from build123d import *

# Parameters (mm, degrees)
F0_R     = 1.5
F1_DEPTH = 2
F2_R     = 1
F3_R     = 1


with BuildPart() as f1:
    # F0 (on Front) → F1 (new body)
    with BuildSketch(Plane.XZ):
        with BuildLine():
            Line((46.64072, -8.883281), (46.64072, 11.116719))
            Line((46.64072, 11.116719), (-24.35928, 11.116719))
            Line((-24.35928, 11.116719), (-24.35928, 1.616719))
            Line((-24.35928, 1.616719), (-8.35928, 1.616719))
            ThreePointArc((-8.35928, 1.616719), (0.64072, 7.25782), (9.64072, 1.616719))
            Line((9.64072, 1.616719), (9.64072, -8.883281))
            Line((9.64072, -8.883281), (46.64072, -8.883281))
        make_face()
        with Locations((42.141477, -3.633281)):
            Circle(F0_R, mode=Mode.SUBTRACT)
        with Locations((-20.358523, 6.366719)):
            Circle(F0_R, mode=Mode.SUBTRACT)
        with Locations((-10.858523, 6.366719)):
            Circle(F0_R, mode=Mode.SUBTRACT)
        with Locations((42.141477, 5.866719)):
            Circle(F0_R, mode=Mode.SUBTRACT)
    extrude(amount=F1_DEPTH)

    # F2
    f2_edges = [f1.edges().sort_by_distance(p)[0] for p in [
        (9.64072, -1, 1.616719),
    ]]
    fillet(f2_edges, radius=F2_R)

    # F3
    f3_edges = [f1.edges().sort_by_distance(p)[0] for p in [
        (46.64072, -1, 11.116719),
        (-24.35928, -1, 11.116719),
        (-24.35928, -1, 1.616719),
        (9.64072, -1, -8.883281),
        (46.64072, -1, -8.883281),
    ]]
    fillet(f3_edges, radius=F3_R)


solid = f1.part
Design review of the part built by this model. Coordinates are the model's own, in mm. A direction names the side the tool comes from. Coordinates: 2 decimals unless noted, no trailing zeros. Write each loop counter-clockwise with the first axis right and the second up, starting at its lowest first coordinate (ties: lowest second). Pieces come first, ordered by that corner, then holes. Notation, with made-up numbers: (51, 24.5) -> (56, 24.5) arc R27 cw to (56, 55.5) -> close; hole circle Ø5 at (-21.75, 4). An arc over 180 degrees is marked (long way). Write each question's results on one line, items separated by ' | '. Start each with the question number.
(1) Tool access review of faces 1 (the face through (-11.18, -0.99, 4.9)), 2 (the face through (9.641, -1, -3)): name each direction out of +Z, -Z, +X, -X, +Y, -Y from which nothing blocks a thin tool from reaching the whole face with its end or side.
(2) Take a section at A-A on y = -1.7. Write out the cut boundary in (x, z), and give its area (3 significant figures).
(3) Take a section at C-C on z = 0.5. Write out the cut boundary in (x, y), and give its area (3 significant figures).
(4) The part is to be moulded in two halves that separate along X. For faces 3 (the face through (19, -2, 3)), 4 (the face through (46.641, -1, 1)), 5 (the face through (43.527, -0.986, 5.292)), say which applies: pulls with the +X half, pulls with the -X half, needs draft (parallel to the pull), parting line crosses it, or undercut.
(5) Take a section at B-B on x = -17. Write out the cut boundary in (y, z).
(6) Clearance check with flat-ended pins moving along their axes: P1, Ø2.5, axis at x = 42.14, z = -3.63, coming from the +Y side; P2, Ø5, axis at x = -20.36, z = 6.37, coming from the +Y side; P3, Ø1, axis at x = -15.5, y = -1, coming from the -Z side. State where each tip first meets the part, or that it passes through.
(7) For line 1 along X through (y, z) = (-0.4, 6.5); line 2 along X through (y, z) = (-0.15, -5.5); line 3 along X through (y, z) = (-1.75, 4.75), list the stretches that pass through material, from the lowest coordinate up. Write a range as from..to.
Results found:
1) face 1: +Y, -Y | face 2: -Z, -X, +Y, -Y
2) outline: (-24.36, 2.62) arc R1 ccw to (-23.36, 1.62) -> (-8.36, 1.62) arc R10 cw to (9.53, 1.84) arc R1 cw to (9.64, 1.38) -> (9.64, -7.88) arc R1 ccw to (10.64, -8.88) -> (45.64, -8.88) arc R1 ccw to (46.64, -7.88) -> (46.64, 10.12) arc R1 ccw to (45.64, 11.12) -> (-23.36, 11.12) arc R1 ccw to (-24.36, 10.12) -> close; hole circle Ø3 at (-20.36, 6.37); hole circle Ø3 at (-10.86, 6.37); hole circle Ø3 at (42.14, -3.63); hole circle Ø3 at (42.14, 5.87) | area: 961 mm2
3) outline: (9.64, -2) -> (46.64, -2) -> (46.64, 0) -> (9.64, 0) -> close | area: 74.0 mm2
4) face 3: needs draft | face 4: pulls with the +X half | face 5: undercut
5) outline: (-2, 1.62) -> (0, 1.62) -> (0, 11.12) -> (-2, 11.12) -> close
6) P1: passes through | P2: stops at y = 0 | P3: stops at z = 1.62
7) line 1: x = -24.36..-21.85, -18.86..-12.35, -9.36..-3.18, 4.46..40.78, 43.5..46.64 | line 2: x = 9.64..46.64 | line 3: x = -24.36..-5.98, 7.26..41.14, 43.14..46.64
